Input: part model. Units: mm. Frame: model coordinates. A direction names the side the tool comes from. Coordinates: 2 decimals unless noted, no trailing zeros. Order: outer loops, then holes, each group sorted by start corner. A loop starts at its lowest first (then second) coordinate and runs counter-clockwise, first axis right, second up. Notation, with made-up numbers: (58, 79) -> (83, 79) arc R18 ccw to (83, 112) -> close; hole circle Ø1 at (86.25, -4.75). An arc over 180 degrees is marked (long way). Use one line per item in the form item = value. Start each with the question number.
1) Access query for faces 1 (the flat face through (42, 10, 39)), 2 (the flat face through (12.809, 7.395, 128.18)), 3 (the flat face through (41, 13, 180)). Directions: +Z, -Z, +X, -X, +Y, -Y. A direction counts if a zero-diameter tool reaches every point of the face in a straight line with its end or side. Return the directions, or none.
2) Section query D-D on y = 3.25. Output: boundary loops of the cut face in (x, z).
3) Ray query, line 1 along X through (y, z) = (12.7, 60); line 2 along X through (y, z) = (13.75, 61); line 3 along Y through (x, z) = (50, 62). Return the intervals inside material, ascending.
4) Draft query along Z for faces 4 (the flat face through (29.9, 10.3, 0)), 5 (the flat face through (41, 15, 70)), 6 (the flat face through (41, 12, 80)). Return one class per face: pulls with the +Z half, pulls with the -Z half, needs draft (parallel to the pull), parting line crosses it, or undercut.
5) Pin query (flat end, axial travel): pin 1 (3 mm diameter, centred on y = 13.5, z = 143.5, fed in from +X); pin 2 (8.5 mm diameter, centred on x = 38.5, z = 234.5, fed in from -Y); pin 3 (1.9 mm diameter, centred on x = 40.98, z = 240, fed in from -Y); pin 4 (3 mm diameter, centred on y = 3, z = 118, fed in from -X). Return the tip coordinate at first contact, or that it passes through.
6) Section query A-A on x = 52.5. Output: boundary loops of the cut face in (y, z).
7) Section query B-B on z = 191.5. Output: boundary loops of the cut face in (x, y), then the cut area to 3 significant figures.
8) Section query C-C on z = 92. Output: boundary loops of the cut face in (x, y), then the cut area to 3 significant figures.
Autodesk Inventor part; units mm, degrees
ref_plane "YZ Plane" through (0, 0, 0) normal (1, 0, 0) x (0, 1, 0)
ref_plane "XZ Plane" through (0, 0, 0) normal (0, 1, 0) x (-1, 0, 0)
ref_plane "XY Plane" through (0, 0, 0) normal (0, 0, 1) x (1, 0, 0)
sketch "スケッチ1" plane through (0, 0, 0) normal (0, 0, 1) x (1, 0, 0)
  line L0 (0, 0) -> (25.9808, 15)
  line L1 (25.9808, 15) -> (55.9808, 15)
  line L2 (55.9808, 15) -> (55.9808, 10)
  line L3 (55.9808, 10) -> (27.3205, 10)
  line L4 (27.3205, 10) -> (10, 0)
  line L5 (10, 0) -> (0, 0)
  dimension "d0" = 15
  dimension "d1" = 5
  dimension "d2" = 5
  dimension "d3" = 30
  dimension "d21" = 30
extrude "押し出し1" add sketch "スケッチ1" along normal blind 260
sketch "スケッチ2" plane through (25.9808, 15, 0) normal (0, 1, 0) x (1, 0, 0)
  line L0 (0.0508, -80) -> (34.0508, -80)
  line L1 (34.0508, -80) -> (34.0508, -180)
  line L2 (34.0508, -180) -> (0.0508, -180)
  line L3 (0.0508, -180) -> (0.0508, -80)
  line L4 (30, 0) -> (0, 0)
  line L5 (30, -260) -> (0, -260)
  point P0 (-25.9808, 0)
  point P1 (15, 0)
  point P2 (17.0508, -180)
  point P3 (15, -260)
  dimension "d7" = 80
  dimension "d8" = 80
  dimension "d22" = 34
extrude "押し出し2" cut sketch "スケッチ2" against normal blind 300
sketch "スケッチ3" plane through (25.9808, 15, 0) normal (0, 1, 0) x (1, 0, 0)
  line L0 (30, 0) -> (30, -260)
  line L1 (30, 0) -> (0, 0)
  line L2 (30, -260) -> (0, -260)
  point P0 (-25.9808, 0)
  point P1 (15, -20)
  point P2 (15, -200)
  point P3 (30, -80)
  point P4 (15, -60)
  point P5 (15, -240)
  point P6 (15, -260)
  dimension "d12" = 15
  dimension "d13" = 20
  dimension "d23" = 40
  dimension "d24" = 20
  dimension "d25" = 40
hole "穴1" at (40.9808, 15, 20) at (40.9808, 15, 200) at (40.9808, 15, 60) at (40.9808, 15, 240) direction (0, -1, 0) diameter 3.2 depth 10 tip angle 118
properties part number "バンパー"
Answers below:
q1.face_1 = +Z, -Z, +X, -Y
q1.face_2 = +Z, -Z, -X, +Y
q1.face_3 = +X, +Y, -Y
q2.outline = (5.63, 0) -> (15.63, 0) -> (15.63, 260) -> (5.63, 260) -> close
q3.line_1 = 22 to 39.38, 42.58 to 55.98
q3.line_2 = 23.82 to 39.73, 42.23 to 55.98
q3.line_3 = 10 to 15
q4.face_4 = pulls with the -Z half
q4.face_5 = needs draft
q4.face_6 = undercut
q5.pin_1 = 26.03
q5.pin_2 = 10
q5.pin_3 = through
q5.pin_4 = 2.6
q6.outline = (10, 0) -> (15, 0) -> (15, 80) -> (10, 80) -> close; (10, 180) -> (15, 180) -> (15, 260) -> (10, 260) -> close
q7.outline = (0, 0) -> (10, 0) -> (27.32, 10) -> (55.98, 10) -> (55.98, 15) -> (25.98, 15) -> close
q7.area = 272 mm^2
q8.outline = (0, 0) -> (10, 0) -> (26.03, 9.26) -> (26.03, 15) -> (25.98, 15) -> close
q8.area = 121 mm^2
